Geometry: final body of the model. Coordinates: model frame, mm. Face numbers are marked on the shaded views. A direction names the side the tool comes from. Round coordinates to 2 decimals unless told otherwise and drop trailing zeros. Loops run counter-clockwise (first coordinate to the right, second up) from the corner with the lowest first, then second, coordinate; pieces in that order, holes last. Notation, with made-up numbers: M 81.25,4.25 L 109.25,4.25 A27 cw 109.25,28.25 Z; hole C 88.5,55.25 d10. An arc over 180 degrees is marked long. Write each question's results on one line, items separated by ' | '.
```python
from build123d import *

# Parameters (mm, degrees)
SKETCH_1_W      = 23
SKETCH_1_H      = 12
EXTRUDE_1_DEPTH = 22
SKETCH_2_W      = 12
SKETCH_2_H      = 2
EXTRUDE_2_DEPTH = 5
SKETCH_3_W      = 5.960545255
SKETCH_3_H      = 1.076312346
EXTRUDE_3_DEPTH = 1.5
SKETCH_4_W      = 12
SKETCH_4_H      = 2
EXTRUDE_4_DEPTH = 5
SKETCH_5_R      = 6.025
EXTRUDE_5_DEPTH = 4
SKETCH_6_R      = 2.5
EXTRUDE_6_DEPTH = 2


with BuildPart() as part:
    # 草图1 → 凸台-拉伸1 (new body)
    with BuildSketch(Plane(origin=(0, 0, 0), x_dir=(1, 0, 0), z_dir=(0, 1, 0))):
        with Locations((11.5, 6)):
            Rectangle(SKETCH_1_W, SKETCH_1_H)
    extrude(amount=EXTRUDE_1_DEPTH)

    # 草图2 → 凸台-拉伸2 (add)
    with BuildSketch(Plane(origin=(23, 0, 0), x_dir=(0, 0, -1), z_dir=(1, 0, 0))):
        with Locations((6, 16)):
            Rectangle(SKETCH_2_W, SKETCH_2_H)
    extrude(amount=EXTRUDE_2_DEPTH)

    # 草图3 → 凸台-拉伸3 (add)
    with BuildSketch(Plane(origin=(23, 0, 0), x_dir=(0, 0, -1), z_dir=(1, 0, 0))):
        with Locations((6.190854898, 4.461843827)):
            Rectangle(SKETCH_3_W, SKETCH_3_H)
    extrude(amount=EXTRUDE_3_DEPTH)

    # 草图4 → 凸台-拉伸4 (add)
    with BuildSketch(Plane.ZY):
        with Locations((-6, 16)):
            Rectangle(SKETCH_4_W, SKETCH_4_H)
    extrude(amount=EXTRUDE_4_DEPTH)

    # 草图5 → 凸台-拉伸5 (add)
    with BuildSketch(Plane(origin=(0, 22, 0), x_dir=(1, 0, 0), z_dir=(0, 1, 0))):
        with Locations(Location((17, 6, 0), (0, 0, 84.778691018))):
            Circle(SKETCH_5_R)
    extrude(amount=EXTRUDE_5_DEPTH)

    # 草图6 → 凸台-拉伸6 (add)
    with BuildSketch(Plane(origin=(0, 26, 0), x_dir=(1, 0, 0), z_dir=(0, 1, 0))):
        with Locations(Location((17, 6, 0), (0, 0, 270))):
            Circle(SKETCH_6_R)
    extrude(amount=EXTRUDE_6_DEPTH)


solid = part.part
```
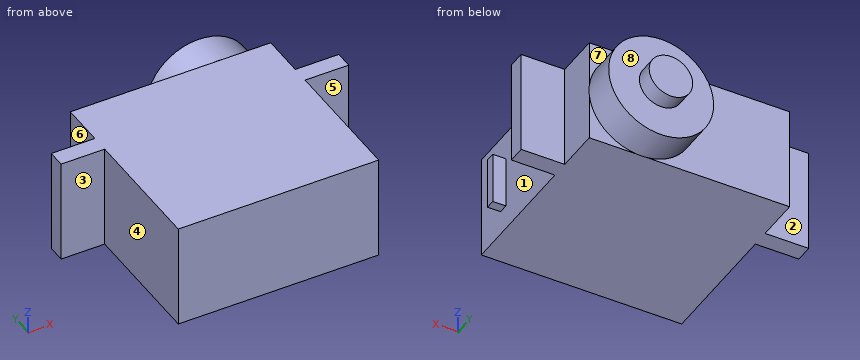
1. Section C-C (y = 3.25). Output: boundary loops of the cut face in (x, z).
Answer key:
outline: M 0,-12 L 23,-12 L 23,0 L 0,0 Z
2. Access query for the marked faces 4, 5, 6, 7 and 8. Directions: +Z, -Z, +X, -X, +Y, -Y. A direction counts if a zero-diameter tool reaches every point of the face in a straight line with its end or side. Return the directions, or none.
Answer key:
face 4: +Z, -Z, -X, -Y | face 5: +Z, -Z, +X | face 6: +Z, -Z, -X, +Y | face 7: +Z, +X, +Y | face 8: +Y
3. Ray query, probe 1 along Y at (x, z) = (-1.5, -8.25); probe 2 along Z at (x, y) = (5.5, 7.25); probe 3 along X at (y, z) = (17.25, -7.75). Return the intervals inside material, ascending.
Answer key:
probe 1: y = 15 to 17 | probe 2: z = -12 to 0 | probe 3: x = 0 to 23
4. Section D-D (z = -2). Output: boundary loops of the cut face in (x, y), then the cut area to 3 significant figures.
Answer key:
outline: M -5,15 L 0,15 L 0,0 L 23,0 L 23,15 L 28,15 L 28,17 L 23,17 L 23,22 L 21.51,22 L 21.51,26 L 12.49,26 L 12.49,22 L 0,22 L 0,17 L -5,17 Z | area: 562 mm²
5. Section A-A (z = -6). Output: boundary loops of the cut face in (x, y) (3 decimals), then the cut area to 3 significant figures.
Answer key:
outline: M -5,15 L 0,15 L 0,0 L 23,0 L 23,3.924 L 24.5,3.924 L 24.5,5 L 23,5 L 23,15 L 28,15 L 28,17 L 23,17 L 23,22 L 23.025,22 L 23.025,26 L 19.5,26 L 19.5,28 L 14.5,28 L 14.5,26 L 10.975,26 L 10.975,22 L 0,22 L 0,17 L -5,17 Z | area: 586 mm²
6. Pin query (flat end, axial travel): P1, Ø1, axis at x = -1.5, y = 19, coming from the -Z side; P2, Ø3.5, axis at y = 9, z = -3, coming from the +X side; P3, Ø4, axis at x = 11, z = -6.5, coming from the +Y side; P4, Ø8, axis at x = 20, y = 9.5, coming from the -Z side. Return the tip coordinate at first contact, or that it passes through.
Answer key:
P1: passes through | P2: stops at x = 23 | P3: stops at y = 26 | P4: stops at z = -12
7. Draft query along Y for the marked faces 1, 2 and 3. Return one class per face: pulls with the +Y half, pulls with the -Y half, needs draft (parallel to the pull), parting line crosses it, or undercut.
Answer key:
face 1: undercut | face 2: pulls with the +Y half | face 3: pulls with the -Y half
8. Section B-B (x = 17). Output: boundary loops of the cut face in (y, z) (3 decimals), then the cut area to 3 significant figures.
Answer key:
outline: M 0,-12 L 22,-12 L 22,-12.025 L 26,-12.025 L 26,-8.5 L 28,-8.5 L 28,-3.5 L 26,-3.5 L 26,0.025 L 22,0.025 L 22,0 L 0,0 Z | area: 322 mm²
